Check sheet for the modelled part. Datum: model origin and axes. Units: mm. A direction names the side the tool comes from. Round coordinates to 2 decimals unless told otherwise and drop trailing zeros. Order: outer loops, then holes, each group sorted by start corner. A loop starts at its lowest first (then second) coordinate and runs counter-clockwise, first axis right, second up.
Q1. Depth check by flat-ended pin: P1, Ø3, axis at x = -10.5, z = 9, coming from the -Y side; P2, Ø8, axis at x = -15, y = 6, coming from the +Z side; P3, Ø4, axis at y = -8, z = 10, coming from the +X side; P4, Ø7, axis at x = 12.5, z = 10, coming from the -Y side. Enter the tip coordinate at first touch or a pass-through.
Q2. Scan lines: probe 1 along X at (y, z) = (3, 17.25); probe 2 along Z at (x, y) = (-12.5, 25.5); probe 3 along Y at (x, z) = (11, 11.75). Record each from-to range of solid material in increasing order.
Q3. Set-up check for faces 4 (the cylindrical face through (17.119, 12.272, 8.085)), 5 (the cylindrical face through (-15.57, -5.05, 9.89)), 6 (the flat face through (-15.5, -8, 10)): record each of +Z, -Z, +X, -X, +Y, -Y from which the full face is reachable in a straight line by a thin tool's end or side.
Q4. Mould release check, pull along X, two halves, no side actions. Record for faces 1 (the cylindrical face through (24.4, 17.25, 19.43)), 2 (the flat face through (-11, 18, 8)), 3 (the flat face through (0, 22, 20)): +X half, -X half, draft (parallel to the pull), parting line (faces both ways), or undercut.
Q5. Cross-section at C-C on x = 0. Record the cut outline in (y, z).
Q6. Cross-section at B-B on z = 10. Give the number of separate pieces and of enclosed holes in the cut face, then the cut area to 3 significant figures.
Q7. Cross-section at A-A on y = 28. Record the cut outline in (x, z).
from build123d import *

# Parameters (mm, degrees)
F1_DEPTH = 20
F3_D     = 4.5
F3_DEPTH = 25
F3_TIP   = 1.3519363928
F6_R     = 2
F5_R     = 5
F7_DEPTH = 15
F8_DEPTH = 10


with BuildPart() as f1:
    # F0 (on Top) → F1 (new body)
    with BuildSketch(Plane.XY):
        with BuildLine():
            ThreePointArc((-15.7857142857, -3.8566467935), (0, 16.25), (15.7857142857, -3.8566467935))
            ThreePointArc((15.7857142857, -3.8566467935), (15.5716855121, -5.0347392879), (15.5, -6.2299678972))
            Line((15.5, -6.2299678972), (15.5, -10.0623058987))
            ThreePointArc((15.5, -10.0623058987), (18.1560750612, -13.4590382547), (22.0930232558, -11.7003556962))
            ThreePointArc((22.0930232558, -11.7003556962), (24.2623739708, -6.0280352771), (25, 0))
            Line((25, 0), (25, 25))
            Line((25, 25), (0, 25))
            Line((0, 25), (-25, 25))
            Line((-25, 25), (-25, 0))
            ThreePointArc((-25, 0), (-24.2623739708, -6.0280352771), (-22.0930232558, -11.7003556962))
            ThreePointArc((-22.0930232558, -11.7003556962), (-18.1560750612, -13.4590382547), (-15.5, -10.0623058987))
            Line((-15.5, -10.0623058987), (-15.5, -6.2299678972))
            ThreePointArc((-15.5, -6.2299678972), (-15.5716855121, -5.0347392879), (-15.7857142857, -3.8566467935))
        make_face()
    extrude(amount=F1_DEPTH)

    # F3
    with Locations(Plane(origin=(0, 25, 0), x_dir=(-1, 0, 0), z_dir=(0, 1, 0))):
        with Locations((-12.5, 10), (12.5, 10)):
            Hole(F3_D / 2, depth=F3_DEPTH)
            with Locations((0, 0, -(F3_DEPTH + F3_TIP / 2))):  # 118° drill point
                Cone(0, F3_D / 2, F3_TIP, mode=Mode.SUBTRACT)

    # F6
    f6_edges = [f1.edges().sort_by_distance(p)[0] for p in [
        (-25, 12.5, 0),
        (-24.262374, -6.028035, 0),
        (0, 16.25, 0),
        (18.156075, -13.459038, 0),
        (25, 12.5, 20),
        (0, 16.25, 20),
        (-18.156075, -13.459038, 20),
    ]]
    fillet(f6_edges, radius=F6_R)

    # F5 (on offset) → F7 (cut)
    with BuildSketch(Plane.XZ.offset(-18)):
        with Locations((-12.5, 10)):
            Circle(F5_R)
        with Locations((12.5, 10)):
            Circle(F5_R)
    extrude(amount=F7_DEPTH, mode=Mode.SUBTRACT)

    # F8 (add): a face of the model
    f8_faces = [f1.faces().sort_by_distance(p)[0] for p in [
        (0, 25, 10),
    ]]
    extrude(f8_faces, amount=F8_DEPTH)


solid = f1.part
Results found:
1. P1: stops at y = 18
1. P2: stops at z = 20
1. P3: stops at x = 24.27
1. P4: stops at y = -11.87
2. probe 1: x = -25 to -15.97, 15.97 to 25
2. probe 2: z = 0 to 7.75, 12.25 to 20
2. probe 3: y = 18 to 35
3. face 4: none
3. face 5: +Z, -Z
3. face 6: +Z, -Z, -Y
4. face 1: +X half
4. face 2: undercut
4. face 3: draft
5. outline: (16.25, 2) arc R2 ccw to (18.25, 0) - (35, 0) - (35, 20) - (18.25, 20) arc R2 ccw to (16.25, 18) - close
6. separate pieces: 3
6. enclosed holes: 0
6. area: 1,220 mm2
7. outline: (-25, 2) arc R2 ccw to (-23, 0) - (23, 0) arc R2 ccw to (25, 2) - (25, 18) arc R2 ccw to (23, 20) - (-23, 20) arc R2 ccw to (-25, 18) - close; hole circle Ø4.5 at (-12.5, 10); hole circle Ø4.5 at (12.5, 10)
